Source: CAD feature listing. Evaluate the final solid. Frame: model axes, mm. A direction names the side the tool comes from. Give positions to 0.01 mm unless a question says otherwise; leave off trailing zeros. Order: outer loops, then holes, each group sorted by start corner. A loop starts at its lowest first (then second) coordinate and runs counter-clockwise, first axis right, second up. Notation, with made-up numbers: (-26.75, 18) - (-1.75, 18) arc R31 cw to (-1.75, 43) - close; hole circle Ø2 at (16.5, 2). An arc over 180 degrees is marked (long way). Answer as CSV lines item,"result".
```python
from build123d import *

# Parameters (mm, degrees)
F1_DEPTH = 3
F2_W     = 2.9827502628
F2_H     = 3
F2_W_2   = 2.9913751314
F2_W_3   = 3
F3_DEPTH = 25


# Not quite as in the source:
# - ends of sketch curves that miss each other by under 0.0002 mm in the source are joined


with BuildPart() as f1:
    # F0 (on Front) → F1 (new body)
    with BuildSketch(Plane.XZ):
        with BuildLine():
            ThreePointArc((-65.4990487043, 31.9219294953), (-59.2590567172, 33.6719294953), (-53.01906473, 31.9219294953))
            Line((-53.01906473, 31.9219294953), (-45.1069841329, 31.9219294953))
            ThreePointArc((-45.1069841329, 31.9219294953), (-45.3487223927, 33.0483271736), (-45.635105941, 34.1642095953))
            ThreePointArc((-45.635105941, 34.1642095953), (-47.0071291889, 38.0195574022), (-48.9092989792, 41.6428024387))
            ThreePointArc((-48.9092989792, 41.6428024387), (-62.9189036621, 37.276531414), (-76.1468158191, 30.9239188806))
            ThreePointArc((-76.1468158191, 30.9239188806), (-84.213049611, 16.9468180053), (-76.0504636415, 3.0257667966))
            ThreePointArc((-76.0504636415, 3.0257667966), (-76.029966864, 3.0142304296), (-76.0094479368, 3.0027335048))
            ThreePointArc((-76.0094479368, 3.0027335048), (-70.4614460946, 1.0953454703), (-64.596721114, 1.2484939552))
            ThreePointArc((-64.596721114, 1.2484939552), (-55.9033559949, 4.8590380101), (-49.1550909719, 11.4219294953))
            Line((-49.1550909719, 11.4219294953), (-53.01906473, 11.4219294953))
            ThreePointArc((-53.01906473, 11.4219294953), (-59.2590567172, 9.6719294953), (-65.4990487043, 11.4219294953))
            Line((-65.4990487043, 11.4219294953), (-67.0090567172, 11.4219294953))
            Line((-67.0090567172, 11.4219294953), (-67.0090567172, 12.5101883944))
            ThreePointArc((-67.0090567172, 12.5101883944), (-71.2590567172, 21.6719294953), (-67.0090567172, 30.8336705962))
            Line((-67.0090567172, 30.8336705962), (-67.0090567172, 31.9219294953))
            Line((-67.0090567172, 31.9219294953), (-65.4990487043, 31.9219294953))
        make_face()
        with BuildLine():
            ThreePointArc((-42.8830074933, 34.1642095953), (-43.1693910416, 33.0483271736), (-43.4111293014, 31.9219294953))
            Line((-43.4111293014, 31.9219294953), (-35.4990487043, 31.9219294953))
            ThreePointArc((-35.4990487043, 31.9219294953), (-29.2590567172, 33.6719294953), (-23.01906473, 31.9219294953))
            Line((-23.01906473, 31.9219294953), (-21.5090567172, 31.9219294953))
            Line((-21.5090567172, 31.9219294953), (-21.5090567172, 30.8336705962))
            ThreePointArc((-21.5090567172, 30.8336705962), (-18.3732861886, 26.7216819645), (-17.2590567172, 21.6719294953))
            ThreePointArc((-17.2590567172, 21.6719294953), (-18.3732861886, 16.6221770261), (-21.5090567172, 12.5101883944))
            Line((-21.5090567172, 12.5101883944), (-21.5090567172, 11.4219294953))
            Line((-21.5090567172, 11.4219294953), (-23.01906473, 11.4219294953))
            ThreePointArc((-23.01906473, 11.4219294953), (-29.2590567172, 9.6719294953), (-35.4990487043, 11.4219294953))
            Line((-35.4990487043, 11.4219294953), (-39.3630224624, 11.4219294953))
            ThreePointArc((-39.3630224624, 11.4219294953), (-32.6147574394, 4.8590380101), (-23.9213923203, 1.2484939552))
            ThreePointArc((-23.9213923203, 1.2484939552), (-18.0566673397, 1.0953454703), (-12.5086654975, 3.0027335048))
            ThreePointArc((-12.5086654975, 3.0027335048), (-12.4881465704, 3.0142304296), (-12.4676497928, 3.0257667966))
            ThreePointArc((-12.4676497928, 3.0257667966), (-4.3050638233, 16.9468180053), (-12.3712976152, 30.9239188806))
            ThreePointArc((-12.3712976152, 30.9239188806), (-25.5992097722, 37.276531414), (-39.6088144552, 41.6428024387))
            ThreePointArc((-39.6088144552, 41.6428024387), (-41.5109842454, 38.0195574022), (-42.8830074933, 34.1642095953))
        make_face()
        with BuildLine():
            Line((-43.5487545967, 21.6719294953), (-44.9693588376, 21.6719294953))
            ThreePointArc((-44.9693588376, 21.6719294953), (-45.3908188129, 19.6558686516), (-45.9763922185, 17.6812209304))
            ThreePointArc((-45.9763922185, 17.6812209304), (-44.2636810752, 17.3202159397), (-42.5729841678, 17.7732590184))
            ThreePointArc((-42.5729841678, 17.7732590184), (-43.1391404553, 19.7030043482), (-43.5487545967, 21.6719294953))
        make_face()
        with BuildLine():
            ThreePointArc((-43.559121813, 21.7346880473), (-43.5539581146, 21.7033054824), (-43.5487545967, 21.6719294953))
            Line((-43.5487545967, 21.6719294953), (-41.2590567172, 21.6719294953))
            ThreePointArc((-41.2590567172, 21.6719294953), (-39.7204118838, 27.550708967), (-35.4990487043, 31.9219294953))
            Line((-35.4990487043, 31.9219294953), (-43.4111293014, 31.9219294953))
            ThreePointArc((-43.4111293014, 31.9219294953), (-43.9370167563, 26.8348735037), (-43.559121813, 21.7346880473))
        make_face()
        with BuildLine():
            ThreePointArc((-53.01906473, 31.9219294953), (-48.7977015505, 27.550708967), (-47.2590567172, 21.6719294953))
            Line((-47.2590567172, 21.6719294953), (-44.9693588376, 21.6719294953))
            ThreePointArc((-44.9693588376, 21.6719294953), (-44.9641553197, 21.7033054824), (-44.9589916213, 21.7346880473))
            ThreePointArc((-44.9589916213, 21.7346880473), (-44.581096678, 26.8348735037), (-45.1069841329, 31.9219294953))
            Line((-45.1069841329, 31.9219294953), (-53.01906473, 31.9219294953))
        make_face()
        with BuildLine():
            Line((-44.9693588376, 21.6719294953), (-47.2590567172, 21.6719294953))
            ThreePointArc((-47.2590567172, 21.6719294953), (-48.7977015505, 15.7931500236), (-53.01906473, 11.4219294953))
            Line((-53.01906473, 11.4219294953), (-49.1550909719, 11.4219294953))
            ThreePointArc((-49.1550909719, 11.4219294953), (-47.3455028522, 14.4397298666), (-45.9763922185, 17.6812209304))
            ThreePointArc((-45.9763922185, 17.6812209304), (-45.3908188129, 19.6558686516), (-44.9693588376, 21.6719294953))
        make_face()
        with BuildLine():
            Line((-41.2590567172, 21.6719294953), (-43.5487545967, 21.6719294953))
            ThreePointArc((-43.5487545967, 21.6719294953), (-43.1391404553, 19.7030043482), (-42.5729841678, 17.7732590184))
            ThreePointArc((-42.5729841678, 17.7732590184), (-41.1945750254, 14.4830849229), (-39.3630224624, 11.4219294953))
            Line((-39.3630224624, 11.4219294953), (-35.4990487043, 11.4219294953))
            ThreePointArc((-35.4990487043, 11.4219294953), (-39.7204118838, 15.7931500236), (-41.2590567172, 21.6719294953))
        make_face()
        with BuildLine():
            ThreePointArc((-44.9589916213, 21.7346880473), (-44.9641553197, 21.7033054824), (-44.9693588376, 21.6719294953))
            Line((-44.9693588376, 21.6719294953), (-43.5487545967, 21.6719294953))
            ThreePointArc((-43.5487545967, 21.6719294953), (-43.5539581146, 21.7033054824), (-43.559121813, 21.7346880473))
            ThreePointArc((-43.559121813, 21.7346880473), (-43.9370167563, 26.8348735037), (-43.4111293014, 31.9219294953))
            Line((-43.4111293014, 31.9219294953), (-45.1069841329, 31.9219294953))
            ThreePointArc((-45.1069841329, 31.9219294953), (-44.581096678, 26.8348735037), (-44.9589916213, 21.7346880473))
        make_face()
        with BuildLine():
            ThreePointArc((-45.635105941, 34.1642095953), (-45.3487223927, 33.0483271736), (-45.1069841329, 31.9219294953))
            Line((-45.1069841329, 31.9219294953), (-43.4111293014, 31.9219294953))
            ThreePointArc((-43.4111293014, 31.9219294953), (-43.1693910416, 33.0483271736), (-42.8830074933, 34.1642095953))
            ThreePointArc((-42.8830074933, 34.1642095953), (-44.2590567172, 34.327758758), (-45.635105941, 34.1642095953))
        make_face()
        with BuildLine():
            Line((-67.0090567172, 11.4219294953), (-65.4990487043, 11.4219294953))
            ThreePointArc((-65.4990487043, 11.4219294953), (-66.2751842679, 11.9367379619), (-67.0090567172, 12.5101883944))
            Line((-67.0090567172, 12.5101883944), (-67.0090567172, 11.4219294953))
        make_face()
        with BuildLine():
            ThreePointArc((-21.5090567172, 12.5101883944), (-22.2429291664, 11.9367379619), (-23.01906473, 11.4219294953))
            Line((-23.01906473, 11.4219294953), (-21.5090567172, 11.4219294953))
            Line((-21.5090567172, 11.4219294953), (-21.5090567172, 12.5101883944))
        make_face()
        with BuildLine():
            Line((-21.5090567172, 31.9219294953), (-23.01906473, 31.9219294953))
            ThreePointArc((-23.01906473, 31.9219294953), (-22.2429291664, 31.4071210287), (-21.5090567172, 30.8336705962))
            Line((-21.5090567172, 30.8336705962), (-21.5090567172, 31.9219294953))
        make_face()
        with BuildLine():
            ThreePointArc((-67.0090567172, 30.8336705962), (-66.2751842679, 31.4071210287), (-65.4990487043, 31.9219294953))
            Line((-65.4990487043, 31.9219294953), (-67.0090567172, 31.9219294953))
            Line((-67.0090567172, 31.9219294953), (-67.0090567172, 30.8336705962))
        make_face()
    extrude(amount=F1_DEPTH)

    # F2 (on face) → F3 (cut)
    with BuildSketch(Plane.XZ.offset(3)):
        Polygon((-67.7719824437, 5.4260265126), (-70.5635935688, 4.3274331729), (-69.4650002292, 1.5358220478), (-66.673389104, 2.6344153875), align=None)
        Polygon((-29.1209643657, 8.7218065315), (-31.9125754908, 9.8203998712), (-33.0111329333, 7.0288799637), (-30.2195218081, 5.930286624), align=None)
        Polygon((-23.5377421156, 6.5246198522), (-26.3293532407, 7.6232131919), (-27.4279286318, 4.8316476756), (-24.6363175066, 3.7330543359), align=None)
        Polygon((-19.0531132051, 1.5358220478), (-17.9545198655, 4.3274331729), (-20.7461309906, 5.4260265126), (-21.8447243303, 2.6344153875), align=None)
        with Locations((-13.8799224838, 9.4239312787)):
            Rectangle(F2_W, F2_H)
        with Locations((-13.8756100495, 15.4239250796)):
            Rectangle(F2_W_2, F2_H)
        with Locations((-13.8712976152, 21.4239188806)):
            Rectangle(F2_W_3, F2_H)
        Polygon((-19.0457892079, 30.3481052815), (-17.9545198238, 33.1211056658), (-20.7461309906, 34.2196988996), (-21.837400333, 31.4466986212), align=None)
        Polygon((-29.120964366, 37.5154789187), (-31.9125754912, 38.6140722584), (-33.0038447503, 35.8410721917), (-30.2122336251, 34.742478852), align=None)
        Polygon((-34.7041866163, 39.712665598), (-37.4957977415, 40.8112589377), (-38.5870669589, 38.0382589769), (-35.7954558337, 36.9396656372), align=None)
        Polygon((-67.7719824437, 34.2196988996), (-70.5635935688, 33.12110556), (-69.4723242264, 30.3481052815), (-66.6807131013, 31.4466986212), align=None)
        Polygon((-55.5142686841, 35.8410721917), (-56.6055380681, 38.614072576), (-59.3971490683, 37.5154789187), (-58.3058798092, 34.742478852), align=None)
        Polygon((-49.9310464754, 38.0382589769), (-51.0223158595, 40.8112593612), (-53.813926818, 39.712665598), (-52.7226576006, 36.9396656372), align=None)
        with Locations((-74.6468158191, 21.4239188806)):
            Rectangle(F2_W_3, F2_H)
        with Locations((-74.6468158191, 9.4239419771)):
            Rectangle(F2_W_3, F2_H)
        Polygon((-61.0901668537, 4.8316020668), (-62.1887601934, 7.623213192), (-64.9803713186, 6.5246198523), (-63.8817779789, 3.7330087272), align=None)
        Polygon((-55.5069446035, 7.0287887462), (-56.6055379431, 9.8203998713), (-59.3971490683, 8.7218065317), (-58.2985557286, 5.9301954065), align=None)
        with Locations((-74.6468158191, 15.4239304289)):
            Rectangle(F2_W_3, F2_H)
    extrude(amount=-F3_DEPTH, mode=Mode.SUBTRACT)


solid = f1.part
```
(1) Ray query, line 1 (X direction, y = -0.6, z = 20); line 2 (X direction, y = -2.7, z = 13.5); line 3 (X direction, y = -2.5, z = 29.5). Return the intervals inside material, ascending. Write a range as from..to.
Completed:
line 1,"-83.93..-76.15, -73.15..-71.14, -47.38..-41.14, -17.38..-15.37, -12.37..-4.59"
line 2,"-83.83..-68.05, -50.47..-47.85, -40.67..-38.05, -20.47..-4.69"
line 3,"-78.23..-68.35, -50.16..-38.35, -20.16..-10.29"
(2) Cut plane C-C (y = -2.25). Give the number of separate pieces and of enclosed holes in the cut face, then the cut area to 3 significant figures.
Completed:
separate pieces,"1"
enclosed holes,"20"
area,"1,280 mm²"
(3) Mould query, pull axis X, two halves, no side actions, for faces 1 (the cylindrical face through (-62.73, -1.48, 37.35)), 2 (the cylindrical face through (-4.308, -1.479, 16.71)), 3 (the flat face through (-62.506, -1.521, 4.275)). Classes: released by +X, released by -X, zero draft, split by the parting line, or undercut.
Completed:
face 1,"released by -X"
face 2,"released by +X"
face 3,"undercut"
(4) Cut plane B-B (x = -75). Return loops of the section in (y, z), then the cut area to 3 significant figures.
Completed:
outline,"(-3, 2.48) - (0, 2.48) - (0, 7.92) - (-3, 7.92) - close; (-3, 10.92) - (0, 10.92) - (0, 13.92) - (-3, 13.92) - close; (-3, 16.92) - (0, 16.92) - (0, 19.92) - (-3, 19.92) - close; (-3, 22.92) - (0, 22.92) - (0, 31.57) - (-3, 31.57) - close"
area,"60.3 mm²"
(5) Cut plane D-D (x = -11.5). Return loops of the section in (y, z).
Completed:
outline,"(-3, 3.62) - (0, 3.62) - (0, 30.39) - (-3, 30.39) - close"
(6) Cut plane A-A (z = 19). Return loops of the section in (x, y).
Completed:
outline,"(-84.09, -3) - (-70.96, -3) - (-70.96, 0) - (-84.09, 0) - close; (-47.56, -3) - (-40.96, -3) - (-40.96, 0) - (-47.56, 0) - close; (-17.56, -3) - (-4.43, -3) - (-4.43, 0) - (-17.56, 0) - close"
(7) Access query for faces 4 (the cylindrical face through (-84.212, -1.479, 17.184)), 5 (the flat face through (-75, -2, 22.924)), 6 (the cylindrical face through (-47, -1, 38)). Directions: +Z, -Z, +X, -X, +Y, -Y. A direction counts if a zero-diameter tool reaches every point of the face in a straight line with its end or side. Return the directions, or none.
Completed:
face 4,"-X, +Y, -Y"
face 5,"+Y, -Y"
face 6,"+Z, +Y, -Y"
(8) Contact query for flat-ended pins moving along their axis: pin 1 (1.5 mm diameter, centred on y = -2, z = 9.5, fed in from -X); pin 2 (0.9 mm diameter, centred on x = -75, y = -1.5, fed in from -Z); pin 3 (1.5 mm diameter, centred on x = -47, y = -2.5, fed in from +Z). Output: stop coordinate, or through.
Completed:
pin 1,"x = -82.72"
pin 2,"z = 2.28"
pin 3,"z = 39.59"
